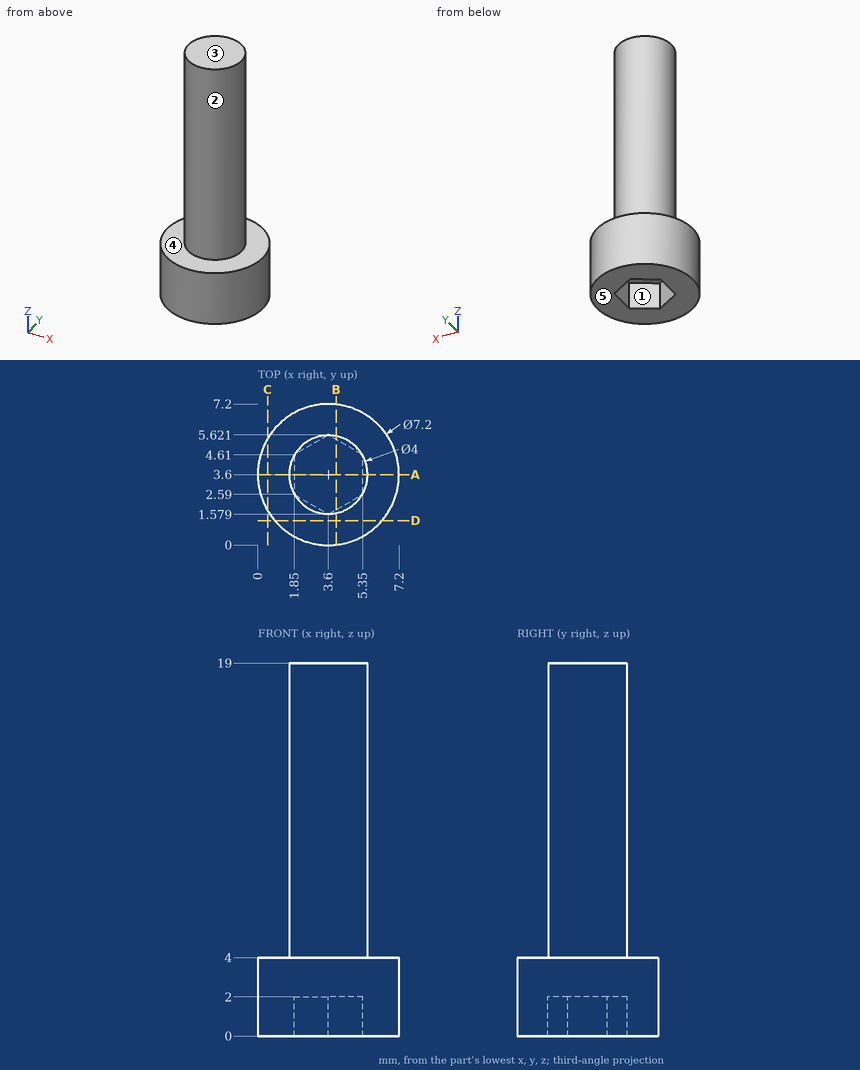
Here's the drawing with two shaded views (mm, measured from the low corner). I have some questions. A direction names the side the tool comes from. Coordinates: 2 decimals unless noted, no trailing zeros. Order: outer loops, then holes, each group sorted by start corner. A loop starts at its lowest first (then second) coordinate and runs counter-clockwise, first axis right, second up.
Q1. Suppose I cut it at B-B on x = 4. Please give me the cut outline in (y, z).
Q2. Suppose I cut it at D-D on y = 1.25. Please give me the cut outline in (x, z).
Q3. Suppose I cut it at A-A on y = 3.6. Please give me the cut outline in (x, z).
Q4. Will these pins go through, and if not, where does the flat tip stop? pin 1 (3 mm diameter, centred on x = 6, z = 7.5, fed in from -Y); pin 2 (3 mm diameter, centred on y = 4.5, z = 7.5, fed in from -X); pin 3 (2 mm diameter, centred on y = 1.5, z = 15, fed in from +X); pin 4 (4 mm diameter, centred on x = 4.5, y = 2.5, fed in from -Z).
Q5. Thinking about a two-plate mould opening in X: for the marked faces 1, 2 and 3, which applies, released by +X, released by -X, zero draft, split by the parting line, or undercut?
Q6. Please list where these lines run through material, in increasing order: L1, parallel to Z at x = 6.5, y = 2.25; L2, parallel to Y at x = 3.5, z = 12.25; L3, parallel to X at y = 3.5, z = 2.75.
Q7. Suppose I cut it at C-C on x = 0.5. Please give me the cut outline in (y, z).
Q8. Which directions (+Z, -Z, +X, -X, +Y, -Y) give clear straight access to the entire face, cutting with the end or side of a thin tool? Please do the marked faces 4 and 5.
Answer:
1. outline: (0.02, 0) - (1.81, 0) - (1.81, 2) - (5.39, 2) - (5.39, 0) - (7.18, 0) - (7.18, 4) - (5.56, 4) - (5.56, 19) - (1.64, 19) - (1.64, 4) - (0.02, 4) - close
2. outline: (0.87, 0) - (6.33, 0) - (6.33, 4) - (0.87, 4) - close
3. outline: (0, 0) - (1.85, 0) - (1.85, 2) - (5.35, 2) - (5.35, 0) - (7.2, 0) - (7.2, 4) - (5.6, 4) - (5.6, 19) - (1.6, 19) - (1.6, 4) - (0, 4) - close
4. pin 1: stops at y = 1.81
4. pin 2: stops at x = 1.6
4. pin 3: stops at x = 5.27
4. pin 4: stops at z = 0
5. face 1: undercut
5. face 2: split by the parting line
5. face 3: zero draft
6. L1: z = 0 to 4
6. L2: y = 1.6 to 5.6
6. L3: x = 0 to 7.2
7. outline: (1.77, 0) - (5.43, 0) - (5.43, 4) - (1.77, 4) - close
8. face 4: +Z
8. face 5: -Z, +X, -X, +Y, -Y
